from build123d import *

# Parameters (mm, degrees)
SKETCH_1_R      = 1.55
EXTRUDE_1_DEPTH = 3
FILLET_1_R      = 15


with BuildPart() as part:
    # 草图1 → 凸台-拉伸1 (new body)
    with BuildSketch(Plane.XY):
        Polygon((0.773502692, 54.641016151), (-25, 10), (-25, -10), (25, -10), (25, 10), (-1.905989232, 10), (18.094010768, 44.641016151), align=None)
        with Locations((-5.56624327, 23.660254038)):
            Circle(SKETCH_1_R, mode=Mode.SUBTRACT)
        with Locations((-1.035875539, 31.507081126)):
            Circle(SKETCH_1_R, mode=Mode.SUBTRACT)
        with Locations((4.43375673, 40.980762114)):
            Circle(SKETCH_1_R, mode=Mode.SUBTRACT)
        with Locations((15, 0)):
            Circle(SKETCH_1_R, mode=Mode.SUBTRACT)
        with Locations((-15, 0)):
            Circle(SKETCH_1_R, mode=Mode.SUBTRACT)
        Circle(SKETCH_1_R, mode=Mode.SUBTRACT)
    extrude(amount=EXTRUDE_1_DEPTH)

    # 圆角1
    fillet_1_edges = [part.edges().sort_by_distance(p)[0] for p in [
        (-1.905989232, 10, 1.5),
    ]]
    fillet(fillet_1_edges, radius=FILLET_1_R)


solid = part.part
Can you work these out from the model? Positions are in its coordinate system, mm. A direction names the side the tool comes from. Round coordinates to 2 decimals unless told otherwise and drop trailing zeros. Write each loop counter-clockwise with the first axis right and the second up, starting at its lowest first coordinate (ties: lowest second). Pieces come first, ordered by that corner, then holes. Notation, with made-up numbers: (69, 50.25) -> (108, 50.25) arc R27 ccw to (108, 72.25) -> close; hole circle Ø9 at (77, 10). An arc over 180 degrees is marked (long way). One line per question, with ' | ' between items. Start each with the question number.
1) Suppose I cut it at D-D on x = -19. Write out the boundary of the cut face in (y, z), then the cut area to 3 significant figures.
2) I'm going to push flat-ended pins straight in: P1, Ø3, axis at x = 3.5, y = -1, coming from the -Z side; P2, Ø0.5, axis at x = 24.5, z = 1.5, coming from the +Y side. Where does each tip first touch, or does it pass through?
3) I need wall thicknesses on line 1 (Y direction, x = 0, z = 1.8); line 2 (Y direction, x = 15, z = 0.6); line 3 (Y direction, x = 12, z = 1.65). Which ranges of each line are inside material? Lowest first, please. Write a range as [from, to].
4) If we mould it in two halves opening along X, with no side actions, what happens to faces 1 (the flat face through (-25, 0, 1)), 2 (the flat face through (0, 16, 3)), 3 (the cylindrical face through (13.45, 0.07, 1.48))? For each: released by +X, released by -X, zero draft, split by the parting line, or undercut.
5) On a 3-axis mill with a long thin cutter (end or side, diameter ignored), from which of +Z, -Z, +X, -X, +Y, -Y can I reach the whole of each face in a straight line? I mean faces 4 (the flat face through (14.54, 38.486, 1.479)), 5 (the flat face through (0, -10, 1)). Say none if no direction works.
6) Suppose I cut it at C-C on x = 15. Write out the boundary of the cut face in (y, z), then the cut area to 3 significant figures.
7) Suppose I cut it at A-A on y = 0. Write out the boundary of the cut face in (x, z), then the cut area to 3 significant figures.
8) Suppose I cut it at B-B on z = 1. Write out the boundary of the cut face in (x, y).
Return value:
1) outline: (-10, 0) -> (20.39, 0) -> (20.39, 3) -> (-10, 3) -> close | area: 91.2 mm2
2) P1: stops at z = 0 | P2: stops at y = 10
3) line 1: y = [-10, -1.55], [1.55, 30.35], [32.66, 53.3] | line 2: y = [-10, -1.55], [1.55, 13.06], [39.28, 46.43] | line 3: y = [-10, 16.1], [34.09, 48.16]
4) face 1: released by -X | face 2: zero draft | face 3: undercut
5) face 4: +Z, -Z, +X | face 5: +Z, -Z, +X, -X, -Y
6) outline: (-10, 0) -> (-1.55, 0) -> (-1.55, 3) -> (-10, 3) -> close; (1.55, 0) -> (13.06, 0) -> (13.06, 3) -> (1.55, 3) -> close; (39.28, 0) -> (46.43, 0) -> (46.43, 3) -> (39.28, 3) -> close | area: 81.3 mm2
7) outline: (-25, 0) -> (-16.55, 0) -> (-16.55, 3) -> (-25, 3) -> close; (-13.45, 0) -> (-1.55, 0) -> (-1.55, 3) -> (-13.45, 3) -> close; (1.55, 0) -> (13.45, 0) -> (13.45, 3) -> (1.55, 3) -> close; (16.55, 0) -> (25, 0) -> (25, 3) -> (16.55, 3) -> close | area: 122 mm2
8) outline: (-25, -10) -> (25, -10) -> (25, 10) -> (24.07, 10) arc R15 cw to (11.08, 32.5) -> (18.09, 44.64) -> (0.77, 54.64) -> (-25, 10) -> close; hole circle Ø3.1 at (-15, 0); hole circle Ø3.1 at (-5.57, 23.66); hole circle Ø3.1 at (-1.04, 31.51); hole circle Ø3.1 at (0, 0); hole circle Ø3.1 at (4.43, 40.98); hole circle Ø3.1 at (15, 0)
